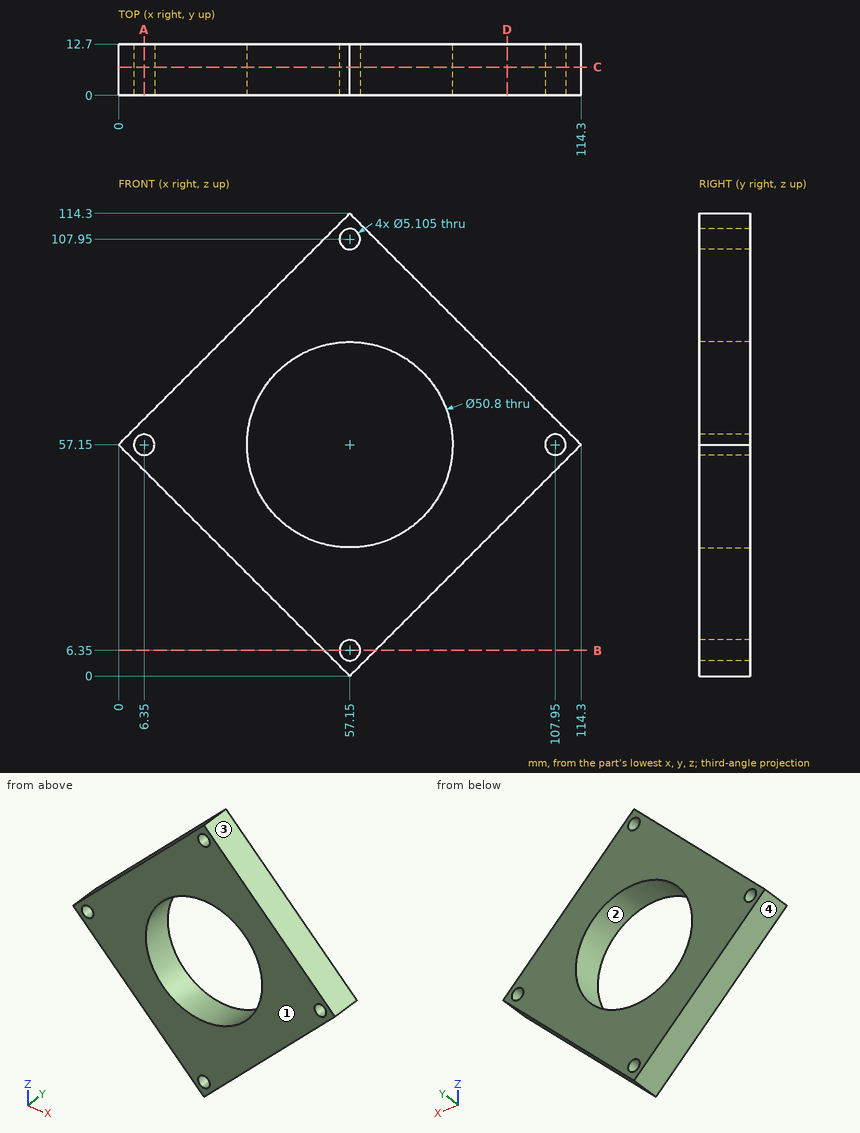
Geometry: see drawing. Coordinates: mm, zero at the bounding-box minimum. Coordinates: 2 decimals unless noted, no trailing zeros. Loops run counter-clockwise (first coordinate to the right, second up) from the corner with the lowest first, then second, coordinate; pieces in that order, holes last.
Q1. Draft query along Z for the marked faces 1, 2, 3 and 4. Return one class per face: +Z half, -Z half, draft (parallel to the pull), parting line (faces both ways), or undercut.
Q2. Cut plane D-D (x = 96). Output: boundary loops of the cut face in (y, z), then the cut area to 3 significant figures.
Q3. Contact query for flat-ended pins moving along their axis: pin 1 (12 mm diameter, centred on x = 14.5, z = 35, fed in from -Y); pin 2 (1 mm diameter, centred on x = 66.5, y = 7, fed in from -Z); pin 3 (6 mm diameter, centred on y = 6.5, z = 53.5, fed in from -X); pin 4 (5 mm diameter, centred on y = 5.5, z = 12.5, fed in from +X). Output: stop coordinate, or through.
Q4. Cut plane C-C (y = 7). Give the number of separate pieces and of enclosed holes in the cut face, then the cut area to 3 significant figures.
Q5. Cut plane B-B (z = 6.35). Output: boundary loops of the cut face in (x, y).
Q6. Cut plane A-A (x = 6.35). Output: boundary loops of the cut face in (y, z).
Q7. Material intervals for line 1 (X direction, y = 7.25, z = 57.5); line 2 (Z direction, x = 57, y = 1); line 3 (X direction, y = 9.75, z = 39), sorted ascending.
Working result:
1. face 1: draft
1. face 2: undercut
1. face 3: +Z half
1. face 4: -Z half
2. outline: (0, 38.85) - (12.7, 38.85) - (12.7, 75.45) - (0, 75.45) - close
2. area: 465 mm2
3. pin 1: stops at y = 0
3. pin 2: stops at z = 8.85
3. pin 3: stops at x = 0.65
3. pin 4: stops at x = 72.15
4. separate pieces: 1
4. enclosed holes: 5
4. area: 4,420 mm2
5. outline: (50.8, 0) - (54.6, 0) - (54.6, 12.7) - (50.8, 12.7) - close; (59.7, 0) - (63.5, 0) - (63.5, 12.7) - (59.7, 12.7) - close
6. outline: (0, 50.8) - (12.7, 50.8) - (12.7, 54.6) - (0, 54.6) - close; (0, 59.7) - (12.7, 59.7) - (12.7, 63.5) - (0, 63.5) - close
7. line 1: x = 0.35 to 3.82, 8.88 to 31.75, 82.55 to 105.42, 110.48 to 113.95
7. line 2: z = 0.15 to 3.8, 8.9 to 31.75, 82.55 to 105.4, 110.5 to 114.15
7. line 3: x = 18.15 to 39.38, 74.92 to 96.15
